Geometry check sheet. Reference: the model listing, model coordinates, mm. A direction names the side the tool comes from. Coordinates: 2 decimals unless noted, no trailing zeros. Write each loop counter-clockwise with the first axis right and the second up, starting at its lowest first coordinate (ties: lowest second). Pieces come first, ordered by that corner, then holes. Notation, with made-up numbers: M 2.25,68 L 52.25,68 A17 cw 52.25,101 Z; hole C 32.5,29.25 d7. An arc over 180 degrees is marked long. Write each question's results on one line, items separated by ' | '.
```python
from build123d import *

# Parameters (mm, degrees)
SKETCH1_W           = 10
SKETCH1_H           = 100.5
SKETCH1_R           = 1.625
SKETCH1_W_2         = 69.85
BOSS_EXTRUDE1_DEPTH = 2
SKETCH3_W           = 149.7
SKETCH3_H           = 2
BOSS_EXTRUDE2_DEPTH = 2
SKETCH4_W           = 100.5
SKETCH4_H           = 2
BOSS_EXTRUDE3_DEPTH = 2
BOSS_EXTRUDE4_DEPTH = 2
SKETCH6_W           = 8
SKETCH6_H           = 15
BOSS_EXTRUDE5_DEPTH = 3
CUT_EXTRUDE1_DEPTH  = 10
FILLET1_R           = 3
CUT_EXTRUDE2_DEPTH  = 10
BOSS_EXTRUDE6_START = 3
SKETCH10_R          = 4
SKETCH10_R_2        = 2.55
BOSS_EXTRUDE6_DEPTH = 3
SKETCH12_R          = 2.875
BOSS_EXTRUDE7_DEPTH = 4
SKETCH13_W          = 10.946886228
SKETCH13_H          = 17.580383234
SKETCH13_W_2        = 10.296538922
SKETCH13_H_2        = 23.433508982
CUT_EXTRUDE3_DEPTH  = 43


with BuildPart() as part:
    # Sketch1 → Boss-Extrude1 (new body)
    # profile 1 of 3: a face of its own
    with BuildSketch(Plane(origin=(0, 0, 0), x_dir=(1, 0, 0), z_dir=(0, 1, 0))):
        with Locations((74.85, 50.25)):
            Rectangle(SKETCH1_W, SKETCH1_H)
    # profile 2 of 3: a face of its own
    with BuildSketch(Plane(origin=(0, 0, 0), x_dir=(1, 0, 0), z_dir=(0, 1, 0))):
        Polygon((0, 0), (69.85, 0), (69.85, 100.5), (0, 100.5), (0, 86.5), align=None)
        with Locations(Location((4.07, 9.9, 0), (0, 0, 270))):
            Circle(SKETCH1_R, mode=Mode.SUBTRACT)
        with BuildLine():
            ThreePointArc((64.165, 9.9), (64.640951481, 11.049048519), (65.79, 11.525))
            ThreePointArc((65.79, 11.525), (66.939048519, 11.049048519), (67.415, 9.9))
            ThreePointArc((67.415, 9.9), (65.79, 8.275), (64.165, 9.9))
        make_face(mode=Mode.SUBTRACT)
        with BuildLine():
            ThreePointArc((5.695, 86.5), (4.07, 84.875), (2.445, 86.5))
            ThreePointArc((2.445, 86.5), (4.07, 88.125), (5.695, 86.5))
        make_face(mode=Mode.SUBTRACT)
        with BuildLine():
            ThreePointArc((65.79, 84.875), (64.640951481, 85.350951481), (64.165, 86.5))
            ThreePointArc((64.165, 86.5), (65.79, 88.125), (67.415, 86.5))
            ThreePointArc((67.415, 86.5), (66.939048519, 85.350951481), (65.79, 84.875))
        make_face(mode=Mode.SUBTRACT)
    # profile 3 of 3: a face of its own
    with BuildSketch(Plane(origin=(0, 0, 0), x_dir=(1, 0, 0), z_dir=(0, 1, 0))):
        with Locations((114.775, 50.25)):
            Rectangle(SKETCH1_W_2, SKETCH1_H)
        with Locations(Location((83.92, 9.9, 0), (0, 0, 270))):
            Circle(SKETCH1_R, mode=Mode.SUBTRACT)
        with Locations(Location((145.64, 9.9, 0), (0, 0, 270))):
            Circle(SKETCH1_R, mode=Mode.SUBTRACT)
        with Locations(Location((83.92, 86.5, 0), (0, 0, 270))):
            Circle(SKETCH1_R, mode=Mode.SUBTRACT)
        with Locations(Location((145.64, 86.5, 0), (0, 0, 270))):
            Circle(SKETCH1_R, mode=Mode.SUBTRACT)
    extrude(amount=BOSS_EXTRUDE1_DEPTH)

    # Sketch3 → Boss-Extrude2 (add)
    with BuildSketch(Plane.XY):
        Polygon((-10, 2), (-10, -13), (159.7, -13), (159.7, 2), (149.7, 2), (149.7, 0), (0, 0), (0, 2), align=None)
        with Locations((74.85, 1)):
            Rectangle(SKETCH3_W, SKETCH3_H)
    extrude(amount=BOSS_EXTRUDE2_DEPTH)

    # Sketch4 → Boss-Extrude3 (add)
    with BuildSketch(Plane.ZY):
        Polygon((0, 0), (-100.5, 0), (0, -13), align=None)
        with Locations((-50.25, 1)):
            Rectangle(SKETCH4_W, SKETCH4_H)
    extrude(amount=BOSS_EXTRUDE3_DEPTH)

    # Sketch5 → Boss-Extrude4 (add)
    with BuildSketch(Plane(origin=(149.7, 0, 0), x_dir=(0, 0, -1), z_dir=(1, 0, 0))):
        Polygon((100.5, 0), (0, -13), (0, 2), (100.5, 2), align=None)
    extrude(amount=BOSS_EXTRUDE4_DEPTH)

    # Sketch6 → Boss-Extrude5 (add)
    with BuildSketch(Plane(origin=(0, 0, 0), x_dir=(-1, 0, 0), z_dir=(0, 0, -1))):
        with Locations((6, -5.5)):
            Rectangle(SKETCH6_W, SKETCH6_H)
        with Locations((-155.7, -5.5)):
            Rectangle(SKETCH6_W, SKETCH6_H)
    extrude(amount=BOSS_EXTRUDE5_DEPTH)

    # Sketch8 → Cut-Extrude1 (cut)
    with BuildSketch(Plane(origin=(0, 0, -3), x_dir=(-1, 0, 0), z_dir=(0, 0, -1))):
        with BuildLine():
            ThreePointArc((-153.15, -5.5), (-155.7, -2.95), (-158.25, -5.5))
            Line((-158.25, -5.5), (-153.15, -5.5))
        make_face()
        with BuildLine():
            Line((-153.15, -5.5), (-158.25, -5.5))
            ThreePointArc((-158.25, -5.5), (-155.7, -8.05), (-153.15, -5.5))
        make_face()
        with BuildLine():
            ThreePointArc((3.45, -5.5), (6, -8.05), (8.55, -5.5))
            Line((8.55, -5.5), (3.45, -5.5))
        make_face()
        with BuildLine():
            Line((3.45, -5.5), (8.55, -5.5))
            ThreePointArc((8.55, -5.5), (6, -2.95), (3.45, -5.5))
        make_face()
    extrude(amount=-CUT_EXTRUDE1_DEPTH, mode=Mode.SUBTRACT)

    # Fillet1
    fillet1_edges = [part.edges().sort_by_distance(p)[0] for p in [
        (159.7, 2, -0.5),
        (-10, 2, -0.5),
        (-10, -13, -0.5),
        (159.7, -13, -0.5),
    ]]
    fillet(fillet1_edges, radius=FILLET1_R)

    # Sketch9 → Cut-Extrude2 (cut)
    with BuildSketch(Plane(origin=(0, 0, 0), x_dir=(-1, 0, 0), z_dir=(0, 0, -1))):
        with BuildLine():
            ThreePointArc((-72.3, -6.5), (-73.046877708, -4.696877708), (-74.85, -3.95))
            Line((-74.85, -3.95), (-74.85, -9.05))
            ThreePointArc((-74.85, -9.05), (-73.046877708, -8.303122292), (-72.3, -6.5))
        make_face()
        with BuildLine():
            Line((-74.85, -9.05), (-74.85, -3.95))
            ThreePointArc((-74.85, -3.95), (-77.4, -6.5), (-74.85, -9.05))
        make_face()
    extrude(amount=-CUT_EXTRUDE2_DEPTH, mode=Mode.SUBTRACT)

    # Sketch10 → Boss-Extrude6 (add)
    with BuildSketch(Plane(origin=(0, 0, 0), x_dir=(-1, 0, 0), z_dir=(0, 0, -1)).offset(BOSS_EXTRUDE6_START)):
        with Locations(Location((-74.85, -6.5, 0), (0, 0, 180))):
            Circle(SKETCH10_R)
        with Locations((-74.85, -6.5)):
            Circle(SKETCH10_R_2, mode=Mode.SUBTRACT)
    extrude(amount=-BOSS_EXTRUDE6_DEPTH)

    # Sketch12 → Boss-Extrude7 (add)
    with BuildSketch(Plane.XY.offset(2)):
        with Locations((34.85, -6.5)):
            Circle(SKETCH12_R)
        with Locations((114.85, -6.5)):
            Circle(SKETCH12_R)
    extrude(amount=BOSS_EXTRUDE7_DEPTH)

    # Sketch13 → Cut-Extrude3 (cut)
    with BuildSketch(Plane(origin=(0, 0, -3), x_dir=(-1, 0, 0), z_dir=(0, 0, -1))):
        with Locations((-157.173443114, -6.790191617)):
            Rectangle(SKETCH13_W, SKETCH13_H)
        with Locations((7.148269461, -9.716754491)):
            Rectangle(SKETCH13_W_2, SKETCH13_H_2)
    extrude(amount=-CUT_EXTRUDE3_DEPTH, mode=Mode.SUBTRACT)


solid = part.part
```
Q1. Depth check by flat-ended pin: P1, Ø1.5, axis at x = 81, z = -10, coming from the -Y side; P2, Ø7.5, axis at x = 65, y = -4, coming from the +Z side; P3, Ø6.5, axis at x = 75.5, y = -6.5, coming from the -Z side. Enter the tip coordinate at first touch or a pass-through.
Geometry check:
P1: stops at y = 0 | P2: stops at z = 2 | P3: stops at z = -3
Q2. Scan lines: probe 1 along X at (y, z) = (0.6, -9.9) (3 decimals); probe 2 along Z at (x, y) = (83.92, 1.15) (3 decimals); probe 3 along X at (y, z) = (-4.25, -66). Record each from-to range of solid material in increasing order.
Geometry check:
probe 1: x = -2 to 2.445, 5.695 to 64.165, 67.415 to 82.295, 85.545 to 144.015, 147.265 to 151.7 | probe 2: z = -100.5 to -88.125, -84.875 to -11.525, -8.275 to 2 | probe 3: x = -2 to 0, 149.7 to 151.7
Q3. Sectioned sample at C-C on z = -21. Record the cut outline in (x, y).
Geometry check:
outline: M -2,-10.28 L 0,-10.28 L 0,0 L 149.7,0 L 149.7,-10.28 L 151.7,-10.28 L 151.7,2 L -2,2 Z
Q4. Sectioned sample at B-B on x = 34.85. Record the cut outline in (y, z) (3 decimals).
Geometry check:
outline: M -13,0 L 0,0 L 0,-100.5 L 2,-100.5 L 2,2 L -3.625,2 L -3.625,6 L -9.375,6 L -9.375,2 L -13,2 Z
Q5. Access from +Z, -Z, +X, -X, +Y, -Y to the whole of each face (thin tool, end or side, straight path). Record for faces 4 (the flat face through (35, -6, 6)), 5 (the cylindrical face through (78.545, -4.968, -1.521)), 6 (the flat face through (0, -4, -29)).
Geometry check:
face 4: +Z, +X, -X, +Y, -Y | face 5: -Z | face 6: -Z, -Y
Q6. Sectioned sample at A-A on x = 145.64. Record the cut outline in (y, z) (3 decimals), and give its area (3 significant figures).
Geometry check:
outline: M -13,0 L 0,0 L 0,-8.275 L 2,-8.275 L 2,2 L -13,2 Z; M 0,-100.5 L 2,-100.5 L 2,-88.125 L 0,-88.125 Z; M 0,-84.875 L 2,-84.875 L 2,-11.525 L 0,-11.525 Z | area: 218 mm2
Q7. Mould release check, pull along Y, two halves, no side actions. Record for faces 1 (the cylindrical face through (36.4, -4.08, 3.97)), 2 (the cylindrical face through (72.6, -7.7, 0)), 3 (the cylindrical face through (82.334, 0.986, -10.252)): pulls with the +Y half, pulls with the -Y half, needs draft (parallel to the pull), parting line crosses it, or undercut.
Geometry check:
face 1: parting line crosses it | face 2: undercut | face 3: needs draft
Q8. Sectioned sample at D-D on x = 17. Record the cut outline in (y, z), and give its area (3 significant figures).
Geometry check:
outline: M -13,0 L 0,0 L 0,-100.5 L 2,-100.5 L 2,2 L -13,2 Z | area: 231 mm2
